Here's how the part is built. I have some questions about the finished solid (model axes, mm). A direction names the side the tool comes from. Coordinates: 2 decimals unless noted, no trailing zeros. Write each loop counter-clockwise with the first axis right and the second up, starting at its lowest first coordinate (ties: lowest second). Pieces come first, ordered by that corner, then holes. Notation, with made-up numbers: (16.25, 35) -> (75.25, 35) arc R15 cw to (75.25, 62) -> close; hole circle Ø10 at (73, 13.25). An arc over 180 degrees is marked (long way). Put each result on its own line as item: value. Start each with the question number.
Item 1: On a 3-axis mill with a long thin cutter (end or side, diameter ignored), from which of +Z, -Z, +X, -X, +Y, -Y can I reach the whole of each face in a straight line? I mean faces 1 (the face through (-12.841, 26, 0)), 2 (the face through (-20.841, 18, 10)), 3 (the face through (-15.841, 17, 0)). Say none if no direction works.
Item 2: I want a section at B-B, the plane z = 16. List the corners of the cut face in (x, y) for me.
Item 3: If we mould it in two halves opening along Y, with no side actions, what happens to faces 4 (the face through (-12.841, 9, 0)), 5 (the face through (-21, 34.447, 6)), 6 (the face through (-21, 2.447, 6)), 7 (the face through (-14, 18.531, 0))? For each: released by +Y, released by -Y, zero draft, split by the parting line, or undercut.
Item 4: For pin 1 (10 mm diameter, centred on y = 18, z = 13.5, fed in from +X); pin 2 (6 mm diameter, centred on x = -15.5, z = 15.5, fed in from -Y); pin 3 (1.6 mm diameter, centred on y = 17.5, z = -0.5, fed in from +X), each with a flat end and sliding along its axis, tell me the tip position at first contact or that it passes through.
Item 5: I need wall thicknesses on line 1 (X direction, y = 27.5, z = 9.5); line 2 (Z direction, x = -14.5, y = 7). Which ranges of each line are inside material? Lowest first, please. Write a range as [from, to].
Item 6: I want a section at A-A, the plane x = -15. List the corners of the cut face in (y, z) for me, then the cut area to 3 significant figures.
Item 7: I want a section at D-D, the plane x = -18.5. List the corners of the cut face in (y, z) for me.
Item 8: I want a section at C-C, the plane y = 20.5. List the corners of the cut face in (x, z) for me, then the cut area to 3 significant figures.
from build123d import *

# Parameters (mm, degrees)
SKETCH034_W     = 10
SKETCH034_H     = 32
PAD018_DEPTH    = 2
SKETCH035_W     = 2
SKETCH035_H     = 32
PAD019_DEPTH    = 20
SKETCH036_W     = 3
SKETCH036_H     = 2.1
POCKET020_DEPTH = 2


with BuildPart() as part:
    # Sketch034 → Pad018 (new body)
    with BuildSketch(Plane.XY):
        with Locations((5, 16)):
            Rectangle(SKETCH034_W, SKETCH034_H)
    extrude(amount=PAD018_DEPTH)

    # Sketch035 (on Face6 of Pad018) → Pad019 (join)
    with BuildSketch(Plane.XY.offset(2)):
        with Locations((1, 16)):
            Rectangle(SKETCH035_W, SKETCH035_H)
    extrude(amount=PAD019_DEPTH)

    # Sketch036 (on Face3 of Pad019) → Pocket020 (cut)
    with BuildSketch(Plane.XY.offset(2)):
        with Locations((8.5, 15.0335876781)):
            Rectangle(SKETCH036_W, SKETCH036_H)
    extrude(amount=-POCKET020_DEPTH, mode=Mode.SUBTRACT)


with BuildPart() as part_1:
    # Body005 placement: moved
    add(part.part.moved(Location((-22.8412186, 2.4472869228, -1.4445826502))))


solid = part_1.part
Calculated:
1. face 1: +Z, -Z, +X, +Y, -Y
1. face 2: +Z, +X, +Y, -Y
1. face 3: +Z, -Z, +X
2. outline: (-22.84, 2.45) -> (-20.84, 2.45) -> (-20.84, 34.45) -> (-22.84, 34.45) -> close
3. face 4: zero draft
3. face 5: released by +Y
3. face 6: released by -Y
3. face 7: undercut
4. pin 1: stops at x = -20.84
4. pin 2: passes through
4. pin 3: stops at x = -15.84
5. line 1: x = [-22.84, -20.84]
5. line 2: z = [-1.44, 0.56]
6. outline: (2.45, -1.44) -> (16.43, -1.44) -> (16.43, 0.56) -> (2.45, 0.56) -> close; (18.53, -1.44) -> (34.45, -1.44) -> (34.45, 0.56) -> (18.53, 0.56) -> close
6. area: 59.8 mm2
7. outline: (2.45, -1.44) -> (34.45, -1.44) -> (34.45, 0.56) -> (2.45, 0.56) -> close
8. outline: (-22.84, -1.44) -> (-12.84, -1.44) -> (-12.84, 0.56) -> (-20.84, 0.56) -> (-20.84, 20.56) -> (-22.84, 20.56) -> close
8. area: 60.0 mm2
